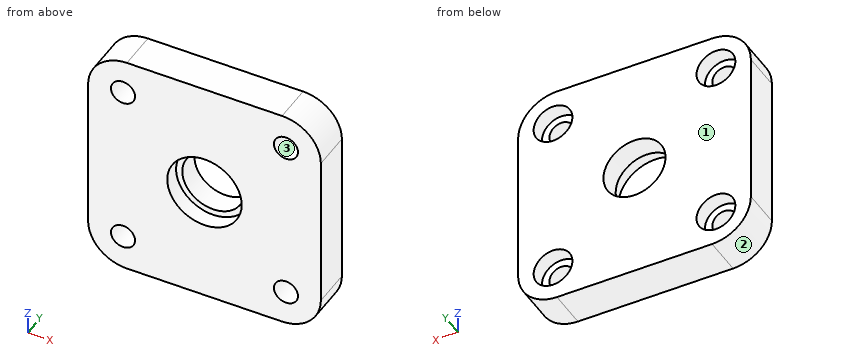
```python
from build123d import *

# Parameters (mm, degrees)
SKETCH1_W               = 30
SKETCH1_H               = 30
BOSS_EXTRUDE1_DEPTH     = 5
SKETCH2_R               = 4
CUT_EXTRUDE1_DEPTH      = 1
CUT_EXTRUDE1_DEPTH_BACK = 6
SKETCH3_R               = 1.55
CUT_EXTRUDE2_DEPTH      = 1
CUT_EXTRUDE2_DEPTH_BACK = 6
SKETCH4_R               = 4.8
CUT_EXTRUDE3_DEPTH      = 2.1
FILLET1_R               = 5
SKETCH5_R               = 2.5
CUT_EXTRUDE4_DEPTH      = 2


with BuildPart() as part:
    # Sketch1 → Boss-Extrude1 (new body)
    with BuildSketch(Plane(origin=(0, 0, 0), x_dir=(1, 0, 0), z_dir=(0, 1, 0))):
        Rectangle(SKETCH1_W, SKETCH1_H)
    extrude(amount=BOSS_EXTRUDE1_DEPTH)

    # Sketch2 → Cut-Extrude1 (cut, two sides)
    with BuildSketch(Plane(origin=(0, 5, 0), x_dir=(1, 0, 0), z_dir=(0, 1, 0))) as cut_extrude1_sk:
        Circle(SKETCH2_R)
    extrude(amount=CUT_EXTRUDE1_DEPTH, mode=Mode.SUBTRACT)
    extrude(cut_extrude1_sk.sketch, amount=-CUT_EXTRUDE1_DEPTH_BACK, mode=Mode.SUBTRACT)

    # Sketch3 → Cut-Extrude2 (cut, two sides)
    with BuildSketch(Plane(origin=(0, 5, 0), x_dir=(1, 0, 0), z_dir=(0, 1, 0))) as cut_extrude2_sk:
        with Locations((-10.5, 10.5)):
            Circle(SKETCH3_R)
        with Locations((10.5, 10.5)):
            Circle(SKETCH3_R)
        with Locations((10.5, -10.5)):
            Circle(SKETCH3_R)
        with Locations((-10.5, -10.5)):
            Circle(SKETCH3_R)
    extrude(amount=CUT_EXTRUDE2_DEPTH, mode=Mode.SUBTRACT)
    extrude(cut_extrude2_sk.sketch, amount=-CUT_EXTRUDE2_DEPTH_BACK, mode=Mode.SUBTRACT)

    # Sketch4 → Cut-Extrude3 (cut)
    with BuildSketch(Plane.XZ):
        Circle(SKETCH4_R)
    extrude(amount=-CUT_EXTRUDE3_DEPTH, mode=Mode.SUBTRACT)

    # Fillet1
    fillet1_edges = [part.edges().sort_by_distance(p)[0] for p in [
        (15, 2.5, 15),
        (-15, 2.5, 15),
        (-15, 2.5, -15),
        (15, 2.5, -15),
    ]]
    fillet(fillet1_edges, radius=FILLET1_R)

    # Sketch5 → Cut-Extrude4 (cut)
    with BuildSketch(Plane(origin=(0, 5, 0), x_dir=(1, 0, 0), z_dir=(0, 1, 0))):
        with Locations((-10.5, 10.5)):
            Circle(SKETCH5_R)
        with Locations((10.5, 10.5)):
            Circle(SKETCH5_R)
        with Locations((-10.5, -10.5)):
            Circle(SKETCH5_R)
        with Locations((10.5, -10.5)):
            Circle(SKETCH5_R)
    extrude(amount=-CUT_EXTRUDE4_DEPTH, mode=Mode.SUBTRACT)


solid = part.part
```
Verification items for the finished model (mm, model axes). Face numbers are marked on the shaded views. Coordinates: 2 decimals unless noted, no trailing zeros. Write each loop counter-clockwise with the first axis right and the second up, starting at its lowest first coordinate (ties: lowest second). Pieces come first, ordered by that corner, then holes. Notation, with made-up numbers: M 31.5,56.5 L 53.5,56.5 A26 ccw 53.5,73.5 Z; hole C -4,67 d9. An arc over 180 degrees is marked long. Answer as a JSON object with one key per item and string values. Group by question number.
(1) Material ranges on line 1 (X direction, y = 0.85, z = 10.75); line 2 (X direction, y = 3.6, z = 10.5); line 3 (Z direction, x = 10.5, y = 1.4), recorded low to high.
(2) Gauge pin test, flat ends, axial feed: pin 1 (3 mm diameter, centred on x = -10.5, z = -10.5, fed in from -Y); pin 2 (2.5 mm diameter, centred on x = -11.5, z = -11, fed in from +Y); pin 3 (1.5 mm diameter, centred on y = 0.5, z = -12, fed in from +X). Record the tip position at first contact, or that the pin passes through.
(3) Cross-section at C-C, the plane x = 10.5. Record the cut outline in (y, z).
(4) Cross-section at D-D, the plane x = -1.75. Record the cut outline in (y, z).
(5) Cross-section at A-A, the plane y = 0.6. Record the cut outline in (x, z), and give its area (3 significant figures).
(6) Release check for a two-part mould opening along Z. For the marked faces 1, 2 and 3 record: +Z half, -Z half, draft (parallel to the pull), parting line (faces both ways), or undercut.
(7) Cross-section at B-B, the plane z = 0. Record the cut outline in (x, y), and give its area (3 significant figures).
Reply:
{
 "1": {"line 1": "-14.94 to -12.03, -8.97 to 8.97, 12.03 to 14.94", "line 2": "-14.97 to -13, -8 to 8, 13 to 14.97", "line 3": "-14.97 to -12.05, -8.95 to 8.95, 12.05 to 14.97"},
 "2": {"pin 1": "through", "pin 2": "y = 3", "pin 3": "x = 14.84"},
 "3": {"outline": "M 0,-14.97 L 5,-14.97 L 5,-13 L 3,-13 L 3,-12.05 L 0,-12.05 Z; M 0,-8.95 L 3,-8.95 L 3,-8 L 5,-8 L 5,8 L 3,8 L 3,8.95 L 0,8.95 Z; M 0,12.05 L 3,12.05 L 3,13 L 5,13 L 5,14.97 L 0,14.97 Z"},
 "4": {"outline": "M 0,-15 L 5,-15 L 5,-3.6 L 2.1,-3.6 L 2.1,-4.47 L 0,-4.47 Z; M 0,4.47 L 2.1,4.47 L 2.1,3.6 L 5,3.6 L 5,15 L 0,15 Z"},
 "5": {"outline": "M -15,-10 A5 ccw -10,-15 L 10,-15 A5 ccw 15,-10 L 15,10 A5 ccw 10,15 L -10,15 A5 ccw -15,10 Z; hole C -10.5,-10.5 d3.1; hole C -10.5,10.5 d3.1; hole C 0,0 d9.6; hole C 10.5,-10.5 d3.1; hole C 10.5,10.5 d3.1", "area": "776 mm²"},
 "6": {"face 1": "draft", "face 2": "-Z half", "face 3": "undercut"},
 "7": {"outline": "M -15,0 L -4.8,0 L -4.8,2.1 L -4,2.1 L -4,5 L -15,5 Z; M 4,2.1 L 4.8,2.1 L 4.8,0 L 15,0 L 15,5 L 4,5 Z", "area": "107 mm²"}
}
